The model under review builds one solid part; all positions refer to its coordinate system, in mm. A direction names the side the tool comes from. Round coordinates to 2 decimals unless told otherwise and drop trailing zeros. Loops run counter-clockwise (first coordinate to the right, second up) from the corner with the lowest first, then second, coordinate; pieces in that order, holes last. Notation, with made-up numbers: (52, 49.5) -> (108, 49.5) arc R26 cw to (108, 74.5) -> close; hole circle Ø1 at (32, 51.25). An arc over 180 degrees is marked (long way). Use a Markdown table: item, result. Add a question column.
1) Consider section A-A on y = -0.3. Give the boundary of the cut face in (x, z) (3 decimals), plus the area to 3 significant figures.
2) For faces 1 (the flat face through (-110.58, -0.78, -184.06)), 2 (the flat face through (-3, 0, -3)), 3 (the flat face through (-110.99, -0.78, 183.65)), list the 3-axis set-ups (+Z, -Z, +X, -X, +Y, -Y) from which the entire face can be reached by the end or side of a thin tool; tool diameter is ignored.
3) Insertion check: pin 1 (6 mm diameter, centred on x = 196.215, z = -154.94, fed in from +Y); pin 2 (0.8 mm diameter, centred on y = -1, z = -179, fed in from +X); pin 3 (0.5 mm diameter, centred on y = -0.5, z = 184.5, fed in from +X). Each pin has a flat end and moves straight along its axis. Give the tip position at first contact, or say it passes through.
4) Wall thickness on probe 1 along X at (y, z) = (-1.2, -0.5); probe 2 along X at (y, z) = (-1, -154.94); probe 3 along X at (y, z) = (-1.2, 180.34): over which ranges is each line inside the solid? List them lowest first.
5) Consider section B-B on x = -108. Give the boundary of the cut face in (y, z).
from build123d import *

# Parameters (mm, degrees)
BOSS_EXTRUDE1_DEPTH   = 1.5875
F_6_CLEARANCE_HOLE1_D = 3.7973
FILLET1_R             = 3.175


with BuildPart() as part:
    # Sketch1 → Boss-Extrude1 (new body)
    with BuildSketch(Plane(origin=(0, 0, 0), x_dir=(1, 0, 0), z_dir=(0, 1, 0))):
        Polygon((199.39, 158.75), (158.75, 199.39), (-95.25, 199.39), (-130.81, 163.83), (-130.81, 199.39), (-199.39, 199.39), (-199.39, -199.39), (-130.81, -199.39), (-130.81, -163.83), (-95.25, -199.39), (158.75, -199.39), (199.39, -158.75), align=None)
    extrude(amount=-BOSS_EXTRUDE1_DEPTH)

    # #6 Clearance Hole1 (through all)
    with Locations(Plane(origin=(0, -1.5875, 0), x_dir=(-1, 0, 0), z_dir=(0, -1, 0))):
        with Locations((196.215, 180.34), (196.215, -180.34), (-196.215, -154.94), (-196.215, 154.94), (196.215, 0), (-196.215, 0)):
            Hole(F_6_CLEARANCE_HOLE1_D / 2)

    # Fillet1
    fillet1_edges = [part.edges().sort_by_distance(p)[0] for p in [
        (-130.81, -0.79375, 199.39),
        (-130.81, -0.79375, -199.39),
        (-130.81, -0.79375, -163.83),
        (-95.25, -0.79375, -199.39),
        (158.75, -0.79375, -199.39),
        (199.39, -0.79375, -158.75),
        (199.39, -0.79375, 158.75),
        (158.75, -0.79375, 199.39),
        (-95.25, -0.79375, 199.39),
        (-130.81, -0.79375, 163.83),
    ]]
    fillet(fillet1_edges, radius=FILLET1_R)


solid = part.part
Result set:
| question | item | result |
|---|---|---|
| 1 | outline | (-199.39, -199.39) -> (-133.985, -199.39) arc R3.175 ccw to (-130.81, -196.215) -> (-130.81, -171.495) arc R3.175 cw to (-125.39, -169.25) -> (-96.18, -198.46) arc R3.175 ccw to (-93.935, -199.39) -> (157.435, -199.39) arc R3.175 ccw to (159.68, -198.46) -> (198.46, -159.68) arc R3.175 ccw to (199.39, -157.435) -> (199.39, 157.435) arc R3.175 ccw to (198.46, 159.68) -> (159.68, 198.46) arc R3.175 ccw to (157.435, 199.39) -> (-93.935, 199.39) arc R3.175 ccw to (-96.18, 198.46) -> (-125.39, 169.25) arc R3.175 cw to (-130.81, 171.495) -> (-130.81, 196.215) arc R3.175 ccw to (-133.985, 199.39) -> (-199.39, 199.39) -> close; hole circle Ø3.797 at (-196.215, -180.34); hole circle Ø3.797 at (-196.215, 0); hole circle Ø3.797 at (-196.215, 180.34); hole circle Ø3.797 at (196.215, -154.94); hole circle Ø3.797 at (196.215, 0); hole circle Ø3.797 at (196.215, 154.94) |
| 1 | area | 156,000 mm2 |
| 2 | face 1 | -Z, +Y, -Y |
| 2 | face 2 | +Z, -Z, +X, -X, +Y |
| 2 | face 3 | +Z, +Y, -Y |
| 3 | pin 1 | y = 0 |
| 3 | pin 2 | x = 179.54 |
| 3 | pin 3 | x = 173.89 |
| 4 | probe 1 | -199.39 to -198.05, -194.38 to 194.38, 198.05 to 199.39 |
| 4 | probe 2 | -199.39 to 194.32, 198.11 to 199.39 |
| 4 | probe 3 | -199.39 to -198.11, -194.32 to -130.81, -114.3 to 177.8 |
| 5 | outline | (-1.59, -186.64) -> (0, -186.64) -> (0, 186.64) -> (-1.59, 186.64) -> close |
